Work out the finished part from the listing and answer in its coordinate system (mm). Face numbers are marked on the shaded views. A direction names the side the tool comes from. Coordinates: 2 decimals unless noted, no trailing zeros. Order: outer loops, then holes, each group sorted by start corner. A loop starts at its lowest first (then second) coordinate and runs counter-clockwise, first axis right, second up. Notation, with made-up numbers: (77, -17.5) -> (97, -17.5) arc R21 ccw to (97, -5.5) -> close; hole circle Ø11 at (63.5, 65.5). An arc over 180 degrees is marked (long way). Answer as CSV lines item,"result". Start each with the question number.
Item 1: Section C-C (x = 0) is taken. Write down the section's boundary in (y, z), then the cut area to 3 significant figures.
Item 2: For a pull along Z with two mould halves and no side action, classify the marked faces 1, 2, 3 and 4 as pulls with the +Z half, pulls with the -Z half, needs draft (parallel to the pull), parting line crosses it, or undercut.
Item 3: Section A-A (y = 6) is taken. Write down the section's boundary in (x, z).
Item 4: Straight lines are drawn through the part: L1, parallel to X at y = 1.2, z = 0; L2, parallel to Y at x = 3.5, z = 9.75; L3, parallel to Z at x = -0.25, y = 4.75. For each, find the intervals that lie inside material, in ascending order.
Item 5: Section B-B (y = 9) is taken. Write down the section's boundary in (x, z), then the cut area to 3 significant figures.
Item 6: Each of these flat-tipped pins is pushed along its axis until it touches: pin 1 Ø1.5 at (x, y) = (11, 7) entering from +Z; pin 2 Ø4 at (x, z) = (5.2, 3) entering from +Y; pin 3 Ø2 at (y, z) = (7, -5) entering from +X. Where does it stop, or does it pass through?
Item 7: Section D-D (z = -3) is taken. Write down the section's boundary in (x, y), then the cut area to 3 significant figures.
Item 8: Which of the six approach directions +Z, -Z, +X, -X, +Y, -Y give full straight-line access (tool end or side, diameter ignored) to the marked faces 5, 6, 7, 8 and 9?
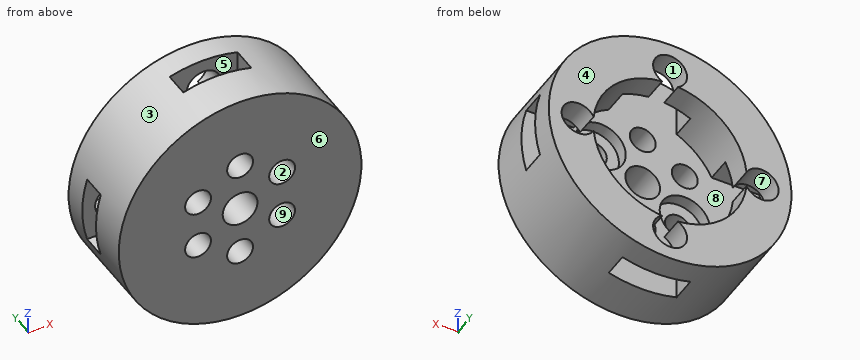
```python
from build123d import *

# Parameters (mm, degrees)
SKETCH1_R           = 10
SKETCH1_R_2         = 1.6
SKETCH1_R_3         = 2.15
BOSS_EXTRUDE1_DEPTH = 5
SKETCH2_R           = 3.1
CUT_EXTRUDE2_DEPTH  = 1.5
SKETCH3_R           = 15
SKETCH3_R_2         = 9.5
BOSS_EXTRUDE2_DEPTH = 11
SKETCH5_R           = 2.1
CUT_EXTRUDE3_DEPTH  = 3
SKETCH7_W           = 10
SKETCH7_H           = 8.4
SKETCH7_W_2         = 8.4
SKETCH7_H_2         = 10
CUT_EXTRUDE4_DEPTH  = 3


with BuildPart() as part:
    # Sketch1 → Boss-Extrude1 (new body)
    with BuildSketch(Plane(origin=(0, 0, 0), x_dir=(1, 0, 0), z_dir=(0, 1, 0))):
        with Locations(Location((0, 0, 0), (0, 0, 270))):
            Circle(SKETCH1_R)
        with Locations(Location((0, 6, 0), (0, 0, 270))):
            Circle(SKETCH1_R_2, mode=Mode.SUBTRACT)
        with Locations(Location((5.196152423, 3, 0), (0, 0, 270))):
            Circle(SKETCH1_R_2, mode=Mode.SUBTRACT)
        with Locations(Location((5.196152423, -3, 0), (0, 0, 270))):
            Circle(SKETCH1_R_2, mode=Mode.SUBTRACT)
        with Locations(Location((0, -6, 0), (0, 0, 270))):
            Circle(SKETCH1_R_2, mode=Mode.SUBTRACT)
        with Locations(Location((-5.196152423, -3, 0), (0, 0, 270))):
            Circle(SKETCH1_R_2, mode=Mode.SUBTRACT)
        with Locations(Location((-5.196152423, 3, 0), (0, 0, 270))):
            Circle(SKETCH1_R_2, mode=Mode.SUBTRACT)
        with Locations(Location((0, 0, 0), (0, 0, 270))):
            Circle(SKETCH1_R_3, mode=Mode.SUBTRACT)
    extrude(amount=BOSS_EXTRUDE1_DEPTH)

    # Sketch2 → Cut-Extrude2 (cut)
    with BuildSketch(Plane(origin=(0, 5, 0), x_dir=(1, 0, 0), z_dir=(0, 1, 0))):
        with Locations(Location((-5.196152423, 3, 0), (0, 0, 270))):
            Circle(SKETCH2_R)
        with Locations(Location((5.196152423, -3, 0), (0, 0, 270))):
            Circle(SKETCH2_R)
    extrude(amount=-CUT_EXTRUDE2_DEPTH, mode=Mode.SUBTRACT)

    # Sketch3 → Boss-Extrude2 (add)
    with BuildSketch(Plane.XZ):
        with Locations(Location((0, 0, 0), (0, 0, 270))):
            Circle(SKETCH3_R)
        with Locations(Location((0, 0, 0), (0, 0, 270))):
            Circle(SKETCH3_R_2, mode=Mode.SUBTRACT)
    extrude(amount=-BOSS_EXTRUDE2_DEPTH)

    # Sketch5 → Cut-Extrude3 (cut)
    with BuildSketch(Plane(origin=(0, 11, 0), x_dir=(1, 0, 0), z_dir=(0, 1, 0))):
        with Locations((0, 11.313708499)):
            Circle(SKETCH5_R)
        with Locations((11.313708499, 0)):
            Circle(SKETCH5_R)
        with Locations((0, -11.313708499)):
            Circle(SKETCH5_R)
        with Locations((-11.313708499, 0)):
            Circle(SKETCH5_R)
    extrude(amount=-CUT_EXTRUDE3_DEPTH, mode=Mode.SUBTRACT)

    # Sketch7 → Cut-Extrude4 (cut)
    with BuildSketch(Plane(origin=(0, 8, 0), x_dir=(1, 0, 0), z_dir=(0, 1, 0))):
        with Locations((-12.313708499, 0)):
            Rectangle(SKETCH7_W, SKETCH7_H)
        with Locations((0, 12.313708499)):
            Rectangle(SKETCH7_W_2, SKETCH7_H_2)
        with Locations((12.313708499, 0)):
            Rectangle(SKETCH7_W, SKETCH7_H)
        with Locations((0, -12.313708499)):
            Rectangle(SKETCH7_W_2, SKETCH7_H_2)
    extrude(amount=-CUT_EXTRUDE4_DEPTH, mode=Mode.SUBTRACT)


solid = part.part
```
Checked values:
1,outline,"(0, -15) -> (5, -15) -> (5, -7.6) -> (0, -7.6) -> close; (0, -4.4) -> (5, -4.4) -> (5, -2.15) -> (0, -2.15) -> close; (0, 2.15) -> (5, 2.15) -> (5, 4.4) -> (0, 4.4) -> close; (0, 7.6) -> (5, 7.6) -> (5, 15) -> (0, 15) -> close; (8, -15) -> (11, -15) -> (11, -13.41) -> (8, -13.41) -> close; (8, 13.41) -> (11, 13.41) -> (11, 15) -> (8, 15) -> close"
1,area,"106 mm^2"
2,face 1,"undercut"
2,face 2,"undercut"
2,face 3,"parting line crosses it"
2,face 4,"needs draft"
3,outline,"(-14.4, -4.2) arc R15 ccw to (-4.2, -14.4) -> (-4.2, -8.52) arc R9.5 cw to (-8.52, -4.2) -> close; (-14.4, 4.2) -> (-8.52, 4.2) arc R9.5 cw to (-4.2, 8.52) -> (-4.2, 14.4) arc R15 ccw to start; (4.2, -14.4) arc R15 ccw to (14.4, -4.2) -> (8.52, -4.2) arc R9.5 cw to (4.2, -8.52) -> close; (4.2, 8.52) arc R9.5 cw to (8.52, 4.2) -> (14.4, 4.2) arc R15 ccw to (4.2, 14.4) -> close"
4,L1,"x = -15 to -2.15, 2.15 to 15"
4,L2,"y = 0 to 5, 8 to 11"
4,L3,"z = -15 to -7.58, -4.42 to -2.14, 2.14 to 4.42, 7.58 to 15"
5,outline,"circle Ø30 at (0, 0); hole (-9.45, -0.97) arc R9.5 ccw to (-0.97, -9.45) arc R2.1 ccw (long way) to (0.97, -9.45) arc R9.5 ccw to (9.45, -0.97) arc R2.1 ccw (long way) to (9.45, 0.97) arc R9.5 ccw to (0.97, 9.45) arc R2.1 ccw (long way) to (-0.97, 9.45) arc R9.5 ccw to (-9.45, 0.97) arc R2.1 ccw (long way) to start"
5,area,"369 mm^2"
6,pin 1,"stops at z = 10.95"
6,pin 2,"stops at y = 3.5"
6,pin 3,"stops at x = 14.4"
7,outline,"(-14.7, 0) -> (-6.8, 0) -> (-6.8, 3.5) -> (-8.3, 3.5) -> (-8.3, 5) -> (-14.7, 5) -> close; (-14.7, 8) -> (-9.01, 8) -> (-9.01, 11) -> (-14.7, 11) -> close; (-3.6, 0) -> (3.6, 0) -> (3.6, 5) -> (-2.1, 5) -> (-2.1, 3.5) -> (-3.6, 3.5) -> close; (6.8, 0) -> (14.7, 0) -> (14.7, 5) -> (6.8, 5) -> close; (9.01, 8) -> (14.7, 8) -> (14.7, 11) -> (9.01, 11) -> close"
7,area,"145 mm^2"
8,face 5,"+Z, -Z"
8,face 6,"+Z, -Z, +X, -X, -Y"
8,face 7,"+Y"
8,face 8,"none"
8,face 9,"+Y, -Y"
